```python
from build123d import *

# Parameters (mm, degrees)
F0_R     = 12.5
F1_DEPTH = 4
F2_R     = 7.35
F3_DEPTH = 10
F4_R     = 1.5
F5_DEPTH = 14.001
F6_R     = 4


with BuildPart() as f1:
    # F0 (on Top) → F1 (new body)
    with BuildSketch(Plane.XY):
        Circle(F0_R)
    extrude(amount=F1_DEPTH)

    # F2 (on face) → F3 (join)
    with BuildSketch(Plane.XY.offset(4)):
        Circle(F2_R)
    extrude(amount=F3_DEPTH)

    # F4 (on face) → F5 (cut, through all)
    with BuildSketch(Plane.XY.offset(14)):
        Circle(F4_R)
    extrude(amount=-F5_DEPTH, mode=Mode.SUBTRACT)

    # F6
    f6_edges = [f1.edges().sort_by_distance(p)[0] for p in [
        (-7.35, 0, 14),
    ]]
    fillet(f6_edges, radius=F6_R)


solid = f1.part
```
Here's how the part is built. I have some questions about the finished solid (model axes, mm). A direction names the side the tool comes from. Give positions to 0.01 mm unless a question says otherwise; leave off trailing zeros. Write each loop counter-clockwise with the first axis right and the second up, starting at its lowest first coordinate (ties: lowest second). Pieces come first, ordered by that corner, then holes. Notation, with made-up numbers: (68.25, 77.5) -> (110.25, 77.5) arc R26 cw to (110.25, 93.5) -> close; hole circle Ø11 at (-24.75, 85). An arc over 180 degrees is marked (long way). Use one line per item in the form item = value.
1) Suppose I cut it at D-D (z = 8.5). Please give me the cut outline in (x, y), and give its area (3 significant figures).
Verdict:
outline = circle Ø14.7 at (0, 0); hole circle Ø3 at (0, 0)
area = 163 mm2
2) Suppose I cut it at A-A (z = 1.5). Please give me the cut outline in (x, y), and give its area (3 significant figures).
Verdict:
outline = circle Ø25 at (0, 0); hole circle Ø3 at (0, 0)
area = 484 mm2
3) We'd pull the mould along X, two halves only. Please class faces 3 (the face through (-1.5, 0.07, 7.1)), 4 (the face through (11.923, 3.755, 1.972)), 5 (the face through (5.4, -5.4, 4)): +X half, -X half, draft (parallel to the pull), parting line (faces both ways), or undercut.
Verdict:
face_3 = undercut
face_4 = parting line
face_5 = draft
4) I'm going to push flat-ended pins straight in: pin 1 (8 mm diameter, centred on x = 1.5, z = 9.5, fed in from +Y); pin 2 (1 mm diameter, centred on y = 1, z = 3.5, fed in from +X); pin 3 (6 mm diameter, centred on y = -4, z = 7.5, fed in from +X). Where does each tip first touch, or does it pass through?
Verdict:
pin_1 = 7.35
pin_2 = 12.49
pin_3 = 7.28
5) On a 3-axis mill with a long thin cutter (end or side, diameter ignored), from which of +Z, -Z, +X, -X, +Y, -Y can I reach the whole of each face in a straight line? I mean faces 1 (the face through (-1.593, -7.175, 6.958)), 2 (the face through (-2, 0, 14)). Say none if no direction works.
Verdict:
face_1 = +Z
face_2 = +Z, +X, -X, +Y, -Y
6) If I drill on L1, parallel to Y at x = 0, z = 6.5; L2, parallel to Z at x = 6.25, y = -4.75; L3, parallel to Y at x = 1, z = 9.5, over which ranges is the centre line in solid material (lowest first)? Write a range as [from, to].
Verdict:
L1 = [-7.35, -1.5], [1.5, 7.35]
L2 = [0, 4]
L3 = [-7.28, -1.12], [1.12, 7.28]
7) Suppose I cut it at B-B (y = -10). Please give me the cut outline in (x, z), and give its area (3 significant figures).
Verdict:
outline = (-7.5, 0) -> (7.5, 0) -> (7.5, 4) -> (-7.5, 4) -> close
area = 60.0 mm2
8) Suppose I cut it at C-C (x = 9). Please give me the cut outline in (y, z), and give its area (3 significant figures).
Verdict:
outline = (-8.67, 0) -> (8.67, 0) -> (8.67, 4) -> (-8.67, 4) -> close
area = 69.4 mm2
